from build123d import *

# Parameters (mm, degrees)
F0_W     = 137.16
F0_H     = 66.04
F0_W_2   = 12.7
F0_H_2   = 12.7
F0_W_3   = 8.89
F0_H_3   = 8.89
F0_R     = 6.35
F1_DEPTH = 50.8
F2_DEPTH = 2.54
F4_DEPTH = 149.098


with BuildPart() as f1:
    # F0 (on Top) → F1 (new body)
    with BuildSketch(Plane.XY):
        with Locations((3.81, -19.05)):
            Rectangle(F0_W, F0_H)
        with Locations((-50.8, -38.1)):
            Rectangle(F0_W_2, F0_H_2, mode=Mode.SUBTRACT)
        with Locations((-31.75, -38.1)):
            Rectangle(F0_W_2, F0_H_2, mode=Mode.SUBTRACT)
        with Locations((-12.7, -38.1)):
            Rectangle(F0_W_2, F0_H_2, mode=Mode.SUBTRACT)
        with Locations((4.445, -40.005)):
            Rectangle(F0_W_3, F0_H_3, mode=Mode.SUBTRACT)
        with Locations((17.145, -40.005)):
            Rectangle(F0_W_3, F0_H_3, mode=Mode.SUBTRACT)
        with Locations((29.845, -40.005)):
            Rectangle(F0_W_3, F0_H_3, mode=Mode.SUBTRACT)
        with Locations((42.545, -40.005)):
            Rectangle(F0_W_3, F0_H_3, mode=Mode.SUBTRACT)
        with Locations((58.42, -38.608)):
            Circle(F0_R, mode=Mode.SUBTRACT)
        with Locations((4.445, -26.035)):
            Rectangle(F0_W_3, F0_H_3, mode=Mode.SUBTRACT)
        with Locations((17.145, -26.035)):
            Rectangle(F0_W_3, F0_H_3, mode=Mode.SUBTRACT)
        with Locations((29.845, -26.035)):
            Rectangle(F0_W_3, F0_H_3, mode=Mode.SUBTRACT)
        with Locations((42.545, -26.035)):
            Rectangle(F0_W_3, F0_H_3, mode=Mode.SUBTRACT)
        with Locations((58.42, -19.304)):
            Circle(F0_R, mode=Mode.SUBTRACT)
        with Locations((-50.8, -19.05)):
            Rectangle(F0_W_2, F0_H_2, mode=Mode.SUBTRACT)
        with Locations((-31.75, -19.05)):
            Rectangle(F0_W_2, F0_H_2, mode=Mode.SUBTRACT)
        with Locations((-12.7, -19.05)):
            Rectangle(F0_W_2, F0_H_2, mode=Mode.SUBTRACT)
        with Locations((-50.8, 0)):
            Rectangle(F0_W_2, F0_H_2, mode=Mode.SUBTRACT)
        with Locations((-31.75, 0)):
            Rectangle(F0_W_2, F0_H_2, mode=Mode.SUBTRACT)
        with Locations((-12.7, 0)):
            Rectangle(F0_W_2, F0_H_2, mode=Mode.SUBTRACT)
        with Locations((4.445, -12.065)):
            Rectangle(F0_W_3, F0_H_3, mode=Mode.SUBTRACT)
        with Locations((17.145, -12.065)):
            Rectangle(F0_W_3, F0_H_3, mode=Mode.SUBTRACT)
        with Locations((29.845, -12.065)):
            Rectangle(F0_W_3, F0_H_3, mode=Mode.SUBTRACT)
        with Locations((42.545, -12.065)):
            Rectangle(F0_W_3, F0_H_3, mode=Mode.SUBTRACT)
        with Locations((4.445, 1.905)):
            Rectangle(F0_W_3, F0_H_3, mode=Mode.SUBTRACT)
        with Locations((17.145, 1.905)):
            Rectangle(F0_W_3, F0_H_3, mode=Mode.SUBTRACT)
        with Locations((29.845, 1.905)):
            Rectangle(F0_W_3, F0_H_3, mode=Mode.SUBTRACT)
        with Locations((42.545, 1.905)):
            Rectangle(F0_W_3, F0_H_3, mode=Mode.SUBTRACT)
        with Locations((58.42, 0)):
            Circle(F0_R, mode=Mode.SUBTRACT)
    extrude(amount=F1_DEPTH)

    # F0 (on Top) → F2 (join)
    with BuildSketch(Plane.XY):
        with Locations((-50.8, 0)):
            Rectangle(F0_W_2, F0_H_2)
        with Locations((-31.75, 0)):
            Rectangle(F0_W_2, F0_H_2)
        with Locations((-50.8, -19.05)):
            Rectangle(F0_W_2, F0_H_2)
        with Locations((-31.75, -19.05)):
            Rectangle(F0_W_2, F0_H_2)
        with Locations((-50.8, -38.1)):
            Rectangle(F0_W_2, F0_H_2)
        with Locations((-31.75, -38.1)):
            Rectangle(F0_W_2, F0_H_2)
        with Locations((-12.7, -38.1)):
            Rectangle(F0_W_2, F0_H_2)
        with Locations((-12.7, -19.05)):
            Rectangle(F0_W_2, F0_H_2)
        with Locations((-12.7, 0)):
            Rectangle(F0_W_2, F0_H_2)
        with Locations((4.445, 1.905)):
            Rectangle(F0_W_3, F0_H_3)
        with Locations((4.445, -12.065)):
            Rectangle(F0_W_3, F0_H_3)
        with Locations((4.445, -26.035)):
            Rectangle(F0_W_3, F0_H_3)
        with Locations((4.445, -40.005)):
            Rectangle(F0_W_3, F0_H_3)
        with Locations((17.145, -40.005)):
            Rectangle(F0_W_3, F0_H_3)
        with Locations((17.145, -26.035)):
            Rectangle(F0_W_3, F0_H_3)
        with Locations((17.145, -12.065)):
            Rectangle(F0_W_3, F0_H_3)
        with Locations((17.145, 1.905)):
            Rectangle(F0_W_3, F0_H_3)
        with Locations((29.845, 1.905)):
            Rectangle(F0_W_3, F0_H_3)
        with Locations((42.545, 1.905)):
            Rectangle(F0_W_3, F0_H_3)
        with Locations((42.545, -12.065)):
            Rectangle(F0_W_3, F0_H_3)
        with Locations((29.845, -12.065)):
            Rectangle(F0_W_3, F0_H_3)
        with Locations((29.845, -26.035)):
            Rectangle(F0_W_3, F0_H_3)
        with Locations((42.545, -26.035)):
            Rectangle(F0_W_3, F0_H_3)
        with Locations((29.845, -40.005)):
            Rectangle(F0_W_3, F0_H_3)
        with Locations((42.545, -40.005)):
            Rectangle(F0_W_3, F0_H_3)
        with Locations((58.42, -38.608)):
            Circle(F0_R)
        with Locations((58.42, -19.304)):
            Circle(F0_R)
        with Locations((58.42, 0)):
            Circle(F0_R)
    extrude(amount=F2_DEPTH)

    # F3 (on face) → F4 (cut)
    with BuildSketch(Plane(origin=(-64.77, 0, 0), x_dir=(0, -1, 0), z_dir=(-1, 0, 0))):
        Polygon((52.07, 50.8), (-13.97, 50.8), (52.07, 41.841079), align=None)
    extrude(amount=-F4_DEPTH, mode=Mode.SUBTRACT)


solid = f1.part
Model file for the job. Use its own axes, mm. Give positions to 0.01 mm unless a question says otherwise; leave off trailing zeros. Loops run counter-clockwise (first coordinate to the right, second up) from the corner with the lowest first, then second, coordinate; pieces in that order, holes last. Notation, with made-up numbers: (36.5, 59.25) - (77.5, 59.25) arc R7 ccw to (77.5, 70.25) - close; hole circle Ø6 at (89, 36.5). An arc over 180 degrees is marked (long way). Use one line per item in the form item = value.
(1) Cut at B-B (z = 9). Count the separate pieces of the cut face and the enclosed holes in it, then the cut area to 3 significant figures.
Determined:
separate_pieces = 1
enclosed_holes = 28
area = 5,960 mm^2
(2) Cut at D-D (x = 58.42). Give the cut face in (y, z).
Determined:
outline = (-52.07, 0) - (13.97, 0) - (13.97, 50.8) - (6.35, 49.77) - (6.35, 2.54) - (-6.35, 2.54) - (-6.35, 48.04) - (-12.95, 47.15) - (-12.95, 2.54) - (-25.65, 2.54) - (-25.65, 45.42) - (-32.26, 44.53) - (-32.26, 2.54) - (-44.96, 2.54) - (-44.96, 42.81) - (-52.07, 41.84) - close
(3) Cut at A-A (x = 27.5). Give the cut face in (y, z).
Determined:
outline = (-52.07, 0) - (13.97, 0) - (13.97, 50.8) - (6.35, 49.77) - (6.35, 2.54) - (-2.54, 2.54) - (-2.54, 48.56) - (-7.62, 47.87) - (-7.62, 2.54) - (-16.51, 2.54) - (-16.51, 46.67) - (-21.59, 45.98) - (-21.59, 2.54) - (-30.48, 2.54) - (-30.48, 44.77) - (-35.56, 44.08) - (-35.56, 2.54) - (-44.45, 2.54) - (-44.45, 42.87) - (-52.07, 41.84) - close
(4) Drill centre lines: L1, parallel to Y at x = 58.42, z = 13; L2, parallel to X at y = -12.5, z = 28; L3, parallel to Y at x = -17.5, z = 29. Where is each one in solid material? Low to high.
Determined:
L1 = -52.07 to -44.96, -32.26 to -25.65, -12.95 to -6.35, 6.35 to 13.97
L2 = -64.77 to 0, 8.89 to 12.7, 21.59 to 25.4, 34.29 to 38.1, 46.99 to 72.39
L3 = -52.07 to -44.45, -31.75 to -25.4, -12.7 to -6.35, 6.35 to 13.97
(5) Cut at C-C (x = -2). Give the cut face in (y, z).
Determined:
outline = (-52.07, 0) - (13.97, 0) - (13.97, 50.8) - (-52.07, 41.84) - close
(6) Drop flat-ended pins along their axis: P1, Ø1, axis at x = 56, y = -43, coming from the +Z side; P2, Ø7, axis at x = 40.5, y = 0, coming from the +Z side. Give the stop position or say it passes through.
Determined:
P1 = 2.54
P2 = 49.25
(7) Pull direction X, two halves, no side cores. Call faces 1 (the face through (-51, -25.4, 24)), 2 (the face through (4, -12, 2.54)): pulls with the +X half, pulls with the -X half, needs draft (parallel to the pull), parting line crosses it, or undercut.
Determined:
face_1 = undercut
face_2 = undercut
